```python
from build123d import *

# Parameters (mm, degrees)
SKETCH_1_R      = 3.95
SKETCH_1_R_2    = 1.5
SKETCH_1_R_3    = 1
EXTRUDE_1_DEPTH = 3
FILLET_1_R      = 5


with BuildPart() as part:
    # 草图1 → 凸台-拉伸1 (new body)
    with BuildSketch(Plane.XY):
        with BuildLine():
            Line((7, 5.916079783), (7, 30))
            ThreePointArc((7, 30), (0, 37), (-7, 30))
            Line((-7, 30), (-7, 0))
            ThreePointArc((-7, 0), (-4.518480571, -5.346338311), (1.166666667, -6.90209308))
            Line((1.166666667, -6.90209308), (24.5, -2.958039892))
            ThreePointArc((24.5, -2.958039892), (27, 0), (24.5, 2.958039892))
            Line((24.5, 2.958039892), (7, 5.916079783))
        make_face()
        Circle(SKETCH_1_R, mode=Mode.SUBTRACT)
        with Locations((0, 15)):
            Circle(SKETCH_1_R_2, mode=Mode.SUBTRACT)
        with Locations((0, 30)):
            Circle(SKETCH_1_R, mode=Mode.SUBTRACT)
        with Locations((24, 0)):
            Circle(SKETCH_1_R_3, mode=Mode.SUBTRACT)
    extrude(amount=EXTRUDE_1_DEPTH)

    # 圆角1
    fillet_1_edges = [part.edges().sort_by_distance(p)[0] for p in [
        (7, 5.916079783, 1.5),
    ]]
    fillet(fillet_1_edges, radius=FILLET_1_R)


solid = part.part
```
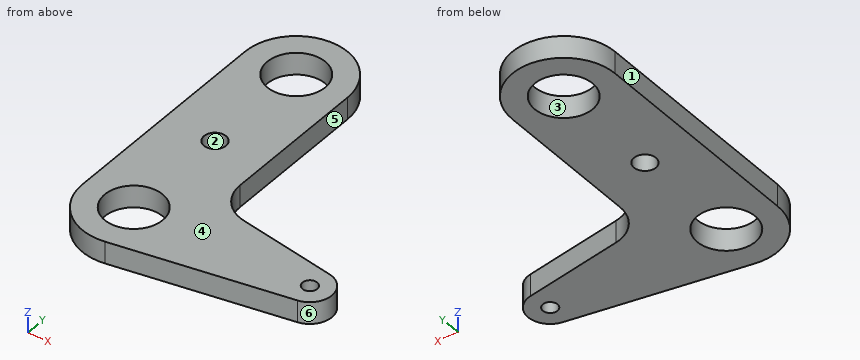
CAD build for the part. Positions are in the model's coordinates, mm. Face numbers are marked on the shaded views. A direction names the side the tool comes from. Round coordinates to 2 decimals unless told otherwise and drop trailing zeros. Write each loop counter-clockwise with the first axis right and the second up, starting at its lowest first coordinate (ties: lowest second). Pieces come first, ordered by that corner, then holes. Notation, with made-up numbers: (30.25, -22) - (69.25, -22) arc R4 cw to (69.25, -17) - close; hole circle Ø1 at (-15, 52.25). An arc over 180 degrees is marked (long way). Return JSON: item names as keys, results as strings. Group by question number.
Item 1: Band-saw the part on B-B on x = 0. List the corners of the cut face in (y, z).
Item 2: 3-axis set-ups, long thin cutter, end or side, ignore diameter. For the marked faces 5 and 6: which of +Z, -Z, +X, -X, +Y, -Y reach the whole face in a straight line?
Item 3: Flat gauge pins, fed straight in: pin 1 Ø1.6 at (x, y) = (24, 0) entering from +Z; pin 2 Ø1.5 at (y, z) = (21.5, 2) entering from +X. Where does each tip first touch, or does it go through?
Item 4: Band-saw the part on C-C on z = 2.1. List the corners of the cut face in (x, y).
Item 5: Band-saw the part on A-A on y = 15. List the corners of the cut face in (x, z).
Item 6: Mould opens along X. For the marked faces 1, 2, 3 and 4 say: +X half, -X half, draft (parallel to the pull), parting line (faces both ways), or undercut.
Item 7: Probe probe 1 along Y at (x, z) = (0, 0.6); probe 2 along Y at (x, z) = (1, 1.55); probe 3 along X at (y, z) = (12, 2). List the from-to ranges inside material, lowest first.
Item 8: Band-saw the part on D-D on x = 24. List the corners of the cut face in (y, z), plus the area to 3 significant figures.
Resolved:
{
 "1": {"outline": "(-7, 0) - (-3.95, 0) - (-3.95, 3) - (-7, 3) - close; (3.95, 0) - (13.5, 0) - (13.5, 3) - (3.95, 3) - close; (16.5, 0) - (26.05, 0) - (26.05, 3) - (16.5, 3) - close; (33.95, 0) - (37, 0) - (37, 3) - (33.95, 3) - close"},
 "2": {"face 5": "+Z, -Z, +X, +Y", "face 6": "+Z, -Z, +X"},
 "3": {"pin 1": "passes through", "pin 2": "stops at x = 7"},
 "4": {"outline": "(-7, 0) arc R7 ccw to (1.17, -6.9) - (24.5, -2.96) arc R3 ccw to (24.5, 2.96) - (11.17, 5.21) arc R5 cw to (7, 10.14) - (7, 30) arc R7 ccw to (-7, 30) - close; hole circle Ø7.9 at (0, 0); hole circle Ø7.9 at (0, 30); hole circle Ø3 at (0, 15); hole circle Ø2 at (24, 0)"},
 "5": {"outline": "(-7, 0) - (-1.5, 0) - (-1.5, 3) - (-7, 3) - close; (1.5, 0) - (7, 0) - (7, 3) - (1.5, 3) - close"},
 "6": {"face 1": "-X half", "face 2": "undercut", "face 3": "undercut", "face 4": "draft"},
 "7": {"probe 1": "y = -7 to -3.95, 3.95 to 13.5, 16.5 to 26.05, 33.95 to 37", "probe 2": "y = -6.93 to -3.82, 3.82 to 13.88, 16.12 to 26.18, 33.82 to 36.93", "probe 3": "x = -7 to 7"},
 "8": {"outline": "(-3.04, 0) - (-1, 0) - (-1, 3) - (-3.04, 3) - close; (1, 0) - (3.04, 0) - (3.04, 3) - (1, 3) - close", "area": "12.3 mm²"}
}
